Verification items for this drawing (mm, ordinates from the low corner). A direction names the side the tool comes from. Round coordinates to 2 decimals unless told otherwise and drop trailing zeros. Loops run counter-clockwise (first coordinate to the right, second up) from the corner with the lowest first, then second, coordinate; pieces in that order, holes last. Notation, with made-up numbers: (62.25, -4) - (77.25, -4) arc R35 ccw to (77.25, 32) - close; hole circle Ø11 at (12, 25). An arc over 180 degrees is marked (long way). Answer in a Markdown table with one row per item. Add a question column.
(1) Cross-section at C-C on x = 14.25. Enter the section's corners in (y, z), then the cut area to 3 significant figures.
(2) Cross-section at D-D on z = 0.5. Enter the section's corners in (x, y), then the cut area to 3 significant figures.
(3) Access from +Z, -Z, +X, -X, +Y, -Y to the whole of each face (thin tool, end or side, straight path). Record for the marked faces 4 and 5.
(4) Cross-section at B-B on x = 3. Enter the section's corners in (y, z).
(5) Mould release check, pull along X, two halves, no side actions. Record for the marked faces 1, 2 and 3: +X half, -X half, draft (parallel to the pull), parting line (faces both ways), or undercut.
(6) Gauge pin test, flat ends, axial feed: pin 1 (3.5 mm diameter, centred on x = 11, y = 6.5, fed in from -Z); pin 2 (3 mm diameter, centred on y = 5.5, z = 4, fed in from +X). Record the tip position at first contact, or that the pin passes through.
(7) Cross-section at A-A on y = 14. Enter the section's corners in (x, z), then the cut area to 3 significant figures.
(8) Thickness scan on line 1 along Y through (x, z) = (3, 4.75); line 2 along X through (y, z) = (5.5, 1.5); line 3 along Z through (x, y) = (11.25, 16.25). Record the ranges inside material, lowest first.
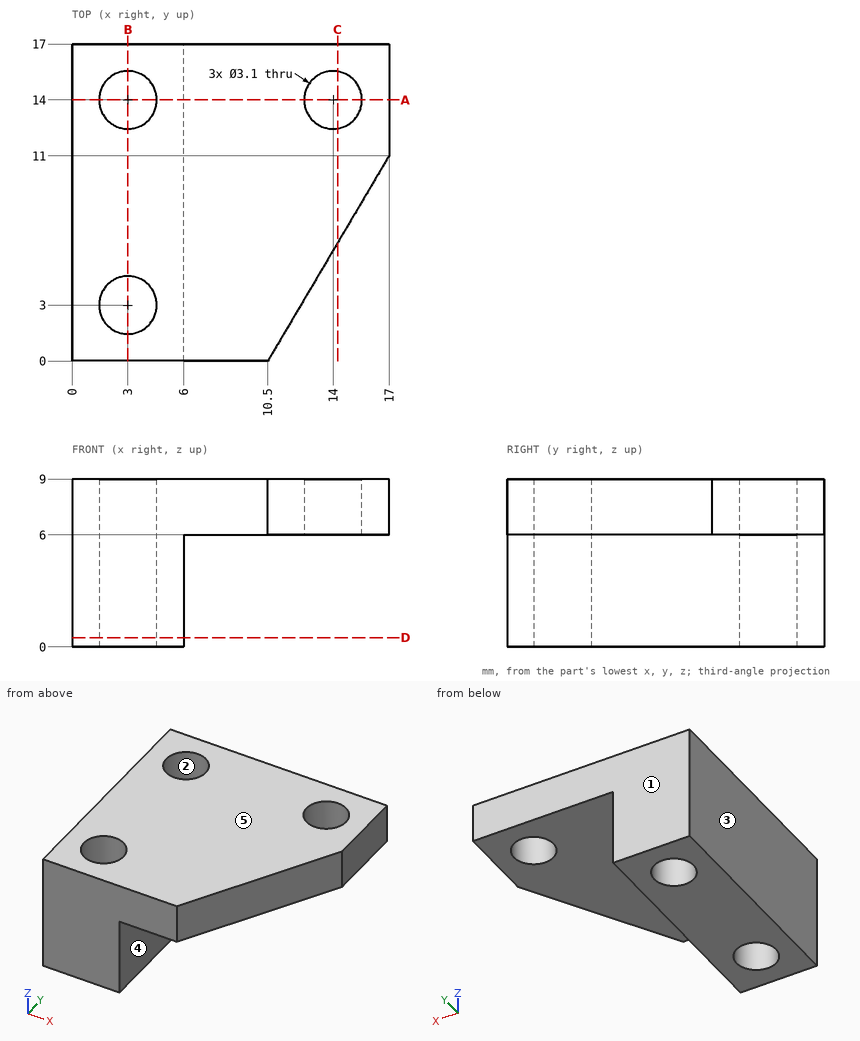
Answers:
| question | item | result |
|---|---|---|
| 1 | outline | (6.35, 6) - (12.47, 6) - (12.47, 9) - (6.35, 9) - close; (15.53, 6) - (17, 6) - (17, 9) - (15.53, 9) - close |
| 1 | area | 22.8 mm^2 |
| 2 | outline | (0, 0) - (6, 0) - (6, 17) - (0, 17) - close; hole circle Ø3.1 at (3, 3); hole circle Ø3.1 at (3, 14) |
| 2 | area | 86.9 mm^2 |
| 3 | face 4 | -Z, +X, +Y, -Y |
| 3 | face 5 | +Z, +X, -X, +Y, -Y |
| 4 | outline | (0, 0) - (1.45, 0) - (1.45, 9) - (0, 9) - close; (4.55, 0) - (12.45, 0) - (12.45, 9) - (4.55, 9) - close; (15.55, 0) - (17, 0) - (17, 9) - (15.55, 9) - close |
| 5 | face 1 | draft |
| 5 | face 2 | undercut |
| 5 | face 3 | -X half |
| 6 | pin 1 | stops at z = 6 |
| 6 | pin 2 | stops at x = 6 |
| 7 | outline | (0, 0) - (1.45, 0) - (1.45, 9) - (0, 9) - close; (4.55, 0) - (6, 0) - (6, 6) - (12.45, 6) - (12.45, 9) - (4.55, 9) - close; (15.55, 6) - (17, 6) - (17, 9) - (15.55, 9) - close |
| 7 | area | 49.8 mm^2 |
| 8 | line 1 | y = 0 to 1.45, 4.55 to 12.45, 15.55 to 17 |
| 8 | line 2 | x = 0 to 6 |
| 8 | line 3 | z = 6 to 9 |
